Part model, mm, in its own coordinate system. Give positions to 0.01 mm unless a question says otherwise; leave off trailing zeros. Write each loop counter-clockwise with the first axis right and the second up, starting at its lowest first coordinate (ties: lowest second). Pieces come first, ordered by that corner, then holes. Notation, with made-up numbers: M 57.25,21 L 71.25,21 A8 cw 71.25,33 Z; hole C 15,26 d3. An arc over 180 degrees is marked long. Answer as CSV lines item,"result". Start each with the question number.
1) Pin check, flat tips, straight feed: pin 1 Ø2 at (x, y) = (-144.5, -55) entering from -Z; pin 2 Ø2 at (y, z) = (48, 10) entering from +X; pin 3 Ø1.5 at (y, z) = (-130, 6.5) entering from +X; pin 4 Ø1.5 at (y, z) = (61.5, 9.5) entering from +X. Stop position of each tip, or through.
2) Mould opens along X. For faces 1 (the cylindrical face through (-17.721, -79.804, 6.409)), 2 (the flat face through (165.07, -97.09, 6.41)), 3 (the flat face through (-2, -191.5, 6)), 4 (the flat face through (-165.07, 97.09, 6.41)) say: pulls with the +X half, pulls with the -X half, needs draft (parallel to the pull), parting line crosses it, or undercut.
3) Slice it at C-C, the plane z = 2.5. Give the cut face in (x, y).
4) Slice it at A-A, the plane x = 95.75. Give the cut face in (y, z), plus the area to 3 significant figures.
5) Slice it at D-D, the plane x = 191.5. Give the cut face in (y, z).
6) Wall check: line 1 along Y through (x, z) = (95.75, 4.5); line 2 along Y through (x, z) = (0, 3); line 3 along X through (y, z) = (-11, 12). Give the ranges that are in metal, low to high. Write a range as from..to.
7) Slice it at B-B, the plane x = 0. Give the cut face in (y, z).
```python
from build123d import *

# Parameters (mm, degrees)
SKETCH_R        = 81.748116
PAD_DEPTH       = 13
SKETCH001_R     = 6
POCKET_DEPTH    = 13.001
SKETCH002_R     = 6
POCKET001_DEPTH = 13.001


with BuildPart() as part:
    # Sketch → Pad (new body)
    with BuildSketch(Plane.XY):
        Polygon((110.562577, 191.5), (-110.562577, 191.5), (-221.125153, 0), (-110.562577, -191.5), (110.562577, -191.5), (221.125153, 0), align=None)
        Circle(SKETCH_R, mode=Mode.SUBTRACT)
    extrude(amount=PAD_DEPTH)

    # Sketch001 (on Face9 of Pad) → Pocket (cut, through all)
    with BuildSketch(Plane.XY.offset(13)):
        with Locations((95.75, 165.843865)):
            Circle(SKETCH001_R)
        with Locations((-95.75, 165.843865)):
            Circle(SKETCH001_R)
        with Locations((-95.75, -165.843865)):
            Circle(SKETCH001_R)
        with Locations((95.75, -165.843865)):
            Circle(SKETCH001_R)
    extrude(amount=-POCKET_DEPTH, mode=Mode.SUBTRACT)

    # Sketch002 (on Face5 of Pocket) → Pocket001 (cut, through all)
    with BuildSketch(Plane.XY.offset(13)):
        with Locations((-191.5, 0)):
            Circle(SKETCH002_R)
        with Locations((191.5, 0)):
            Circle(SKETCH002_R)
    extrude(amount=-POCKET001_DEPTH, mode=Mode.SUBTRACT)


solid = part.part
```
Found:
1,pin 1,"z = 0"
1,pin 2,"x = 193.99"
1,pin 3,"x = 146.5"
1,pin 4,"x = 186.05"
2,face 1,"undercut"
2,face 2,"pulls with the +X half"
2,face 3,"needs draft"
2,face 4,"pulls with the -X half"
3,outline,"M -221.13,0 L -110.56,-191.5 L 110.56,-191.5 L 221.13,0 L 110.56,191.5 L -110.56,191.5 Z; hole C -191.5,0 d12; hole C -95.75,-165.84 d12; hole C -95.75,165.84 d12; hole C 0,0 d163.5; hole C 95.75,-165.84 d12; hole C 95.75,165.84 d12; hole C 191.5,0 d12"
4,outline,"M -191.5,0 L -171.84,0 L -171.84,13 L -191.5,13 Z; M -159.84,0 L 159.84,0 L 159.84,13 L -159.84,13 Z; M 171.84,0 L 191.5,0 L 191.5,13 L 171.84,13 Z"
4,area,"4,670 mm²"
5,outline,"M -51.31,0 L -6,0 L -6,13 L -51.31,13 Z; M 6,0 L 51.31,0 L 51.31,13 L 6,13 Z"
6,line 1,"-191.5..-171.84, -159.84..159.84, 171.84..191.5"
6,line 2,"-191.5..-81.75, 81.75..191.5"
6,line 3,"-214.77..-81, 81..214.77"
7,outline,"M -191.5,0 L -81.75,0 L -81.75,13 L -191.5,13 Z; M 81.75,0 L 191.5,0 L 191.5,13 L 81.75,13 Z"
